Design review of the part built by this model. Coordinates are the model's own, in mm. Face numbers are marked on the shaded views. A direction names the side the tool comes from. Round coordinates to 2 decimals unless told otherwise and drop trailing zeros. Loops run counter-clockwise (first coordinate to the right, second up) from the corner with the lowest first, then second, coordinate; pieces in that order, holes last. Notation, with made-up numbers: (73, 0) - (114, 0) arc R28 cw to (114, 37) - close; hole circle Ø5 at (-12, -3.75). An arc over 180 degrees is marked (long way). Return JSON: item names as keys, results as strings. Group by question number.
from build123d import *

# Parameters (mm, degrees)
F1_DEPTH  = 20
F2_R      = 20
F3_DEPTH  = 30
F4_DEPTH  = 40
F5_W      = 33
F5_H      = 20
F6_DEPTH  = 55
F7_R      = 15
F8_DEPTH  = 20
F9_D      = 20
F11_R     = 25
F12_DEPTH = 70
F13_R     = 5


with BuildPart() as f1:
    # F0 (on Front) → F1 (new body)
    with BuildSketch(Plane.XZ):
        with BuildLine():
            ThreePointArc((-109.5042586091, -28.4546844701), (-82.4661435827, -24.3426350081), (-70, 0))
            ThreePointArc((-70, 0), (-82.4661435827, 24.3426350081), (-109.5042586091, 28.4546844701))
            ThreePointArc((-109.5042586091, 28.4546844701), (-130, 0), (-109.5042586091, -28.4546844701))
        make_face()
        with BuildLine():
            ThreePointArc((-109.5042586091, 28.4546844701), (-82.4661435827, 24.3426350081), (-70, 0))
            ThreePointArc((-70, 0), (-82.4661435827, -24.3426350081), (-109.5042586091, -28.4546844701))
            Line((-109.5042586091, -28.4546844701), (-58.6638275939, -45.4360923882))
            ThreePointArc((-58.6638275939, -45.4360923882), (-48.7715766613, -52.7166444234), (-45, -64.4058820349))
            Line((-45, -64.4058820349), (-45, -130))
            ThreePointArc((-45, -130), (-50.8578643763, -144.1421356237), (-65, -150))
            Line((-65, -150), (-80, -150))
            Line((-80, -150), (-80, -210))
            Line((-80, -210), (-60, -210))
            Line((-60, -210), (-60, -170))
            Line((-60, -170), (60, -170))
            Line((60, -170), (60, -210))
            Line((60, -210), (80, -210))
            Line((80, -210), (80, -150))
            Line((80, -150), (65, -150))
            ThreePointArc((65, -150), (50.8578643763, -144.1421356237), (45, -130))
            Line((45, -130), (45, -64.4058820349))
            ThreePointArc((45, -64.4058820349), (48.7715766613, -52.7166444234), (58.6638275939, -45.4360923882))
            Line((58.6638275939, -45.4360923882), (109.5042586091, -28.4546844701))
            ThreePointArc((109.5042586091, -28.4546844701), (70, 0), (109.5042586091, 28.4546844701))
            Line((109.5042586091, 28.4546844701), (45, 50))
            Line((45, 50), (0, 50))
            Line((0, 50), (-45, 50))
            Line((-45, 50), (-109.5042586091, 28.4546844701))
        make_face()
        with BuildLine():
            ThreePointArc((130, 0), (124.3426350081, 17.5338564173), (109.5042586091, 28.4546844701))
            ThreePointArc((109.5042586091, 28.4546844701), (70, 0), (109.5042586091, -28.4546844701))
            ThreePointArc((109.5042586091, -28.4546844701), (124.3426350081, -17.5338564173), (130, 0))
        make_face()
    extrude(amount=F1_DEPTH)

    # F2 (on face) → F3 (join)
    with BuildSketch(Plane.XZ.offset(20)):
        with Locations((100, 0)):
            Circle(F2_R)
        with Locations((-100, 0)):
            Circle(F2_R)
    extrude(amount=F3_DEPTH)

    # F2 (on face) → F4 (join)
    with BuildSketch(Plane.XZ.offset(20)):
        Polygon((-65, -150), (-80, -150), (-80, -210), (-60, -210), (-60, -170), (60, -170), (60, -210), (80, -210), (80, -150), (65, -150), align=None)
    extrude(amount=F4_DEPTH)

    # F5 (on face) → F6 (join)
    with BuildSketch(Plane.XZ.offset(60)):
        with Locations((16.5, -160)):
            Rectangle(F5_W, F5_H)
        with Locations((-16.5, -160)):
            Rectangle(F5_W, F5_H)
    extrude(amount=F6_DEPTH)

    # F7 (on face) → F8 (join)
    with BuildSketch(Plane.XZ.offset(115)):
        with BuildLine():
            ThreePointArc((-33, -227), (0, -260), (33, -227))
            ThreePointArc((33, -227), (0, -194), (-33, -227))
        make_face()
        with Locations((0, -227)):
            Circle(F7_R, mode=Mode.SUBTRACT)
        with BuildLine():
            ThreePointArc((-33, -227), (0, -194), (33, -227))
            Line((33, -227), (33, -170))
            Line((33, -170), (33, -150))
            Line((33, -150), (-33, -150))
            Line((-33, -150), (-33, -170))
            Line((-33, -170), (-33, -227))
        make_face()
    extrude(amount=F8_DEPTH)

    # F9 (through all)
    with Locations(Plane(origin=(0, 0, 0), x_dir=(1, 0, 0), z_dir=(0, 1, 0))):
        with Locations((100, 0), (-100, 0)):
            Hole(F9_D / 2)

    # F11 (on offset) → F12 (join)
    with BuildSketch(Plane.XY.offset(35)):
        with BuildLine():
            ThreePointArc((-39.9505821476, -78.0122912513), (-0.9941614801, -119.9876436284), (40, -80))
            ThreePointArc((40, -80), (39.9876436284, -79.0058385199), (39.9505821476, -78.0122912513))
            ThreePointArc((39.9505821476, -78.0122912513), (0, -40), (-39.9505821476, -78.0122912513))
        make_face()
        with Locations((0, -80)):
            Circle(F11_R, mode=Mode.SUBTRACT)
        with BuildLine():
            ThreePointArc((-39.9505821476, -78.0122912513), (0, -40), (39.9505821476, -78.0122912513))
            Line((39.9505821476, -78.0122912513), (39.9505821476, -30))
            ThreePointArc((39.9505821476, -30), (42.8795143357, -22.9289321881), (49.9505821476, -20))
            Line((49.9505821476, -20), (-49.9505821476, -20))
            ThreePointArc((-49.9505821476, -20), (-42.8795143357, -22.9289321881), (-39.9505821476, -30))
            Line((-39.9505821476, -30), (-39.9505821476, -78.0122912513))
        make_face()
    extrude(amount=-F12_DEPTH)

    # F13
    f13_edges = [f1.edges().sort_by_distance(p)[0] for p in [
        (-120, -20, 0),
        (80, -20, 0),
    ]]
    fillet(f13_edges, radius=F13_R)


solid = f1.part
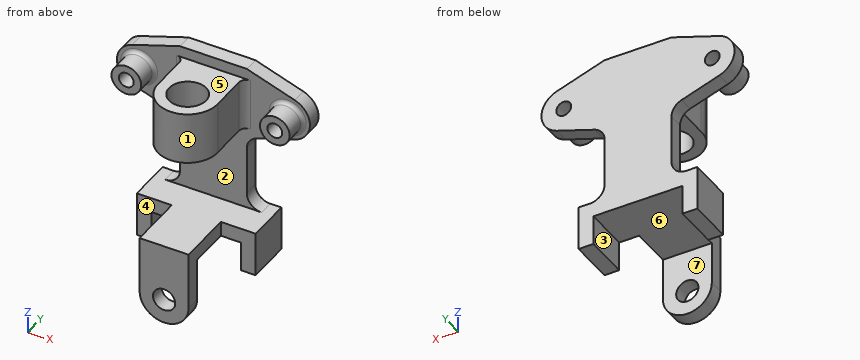
Q1. For line 1 (X direction, y = -17, z = -0.5); line 2 (Z direction, x = 39.5, y = -44.5); line 3 (Y direction, x = 0, z = 9), list the stretches that pass through material, from the lowest coordinate up.
Q2. Add section C-C, the plane x = -100. State the section outline as (y, z) points.
Q3. Add section D-D, the plane z = 4. Give the number of separate pieces and of enclosed holes in the cut face, plus the area to 3 significant figures.
Q4. Add section A-A, the plane z = -174. State the section outline as (x, y) points, plus the area to 3 significant figures.
Q5. Draft analysis for pull direction X (two halves, no side actions). For the marked faces 1, 2, 3 and 4, state which applies: pulls with the +X half, pulls with the -X half, needs draft (parallel to the pull), parting line crosses it, or undercut.
Q6. Add section B-B, the plane x = 0. State the section outline as (y, z) points.
Q7. Insertion check: pin 1 Ø14.5 at (y, z) = (-44.5, 6.5) entering from +X; pin 2 Ø6 at (x, y) = (68, -43.5) entering from -Z; pin 3 Ø3 at (x, z) = (-4.5, -103) entering from -Y. Each pin has a flat end and moves straight along its axis. Give the tip position at first contact, or say it passes through.
Q8. Tool access review of the marked faces 5, 6 and 7: name each direction out of +Z, -Z, +X, -X, +Y, -Y from which nothing blocks a thin tool from reaching the whole face with its end or side.
Evaluation:
{
 "1": {"line 1": "-130 to -109.99, -90.01 to 90.01, 109.99 to 130", "line 2": "-170 to -150, -35 to 35", "line 3": "-120 to -105, -55 to 0"},
 "2": {"outline": "(-50, -20) - (-25, -20) arc R5 cw to (-20, -25) - (-20, -31.63) - (0, -31.63) - (0, -10) - (-50, -10) - close; (-50, 10) - (0, 10) - (0, 31.63) - (-20, 31.63) - (-20, 25) arc R5 cw to (-25, 20) - (-50, 20) - close"},
 "3": {"separate pieces": "3", "enclosed holes": "1", "area": "11,100 mm²"},
 "4": {"outline": "(-80, -60) - (-60, -60) - (-60, 0) - (-80, 0) - close; (-33, -135) - (33, -135) - (33, -115) - (-33, -115) - close; (60, -60) - (80, -60) - (80, 0) - (60, 0) - close", "area": "3,720 mm²"},
 "5": {"face 1": "parting line crosses it", "face 2": "undercut", "face 3": "undercut", "face 4": "needs draft"},
 "6": {"outline": "(-135, -260) - (-115, -260) - (-115, -242) - (-135, -242) - close; (-135, -212) - (-115, -212) - (-115, -170) - (0, -170) - (0, 50) - (-20, 50) - (-20, 35) - (-55, 35) - (-55, -35) - (-20, -35) - (-20, -150) - (-135, -150) - close; (-120, -35) - (-105, -35) - (-105, 35) - (-120, 35) - close"},
 "7": {"pin 1": "x = 120", "pin 2": "z = -210", "pin 3": "y = -20"},
 "8": {"face 5": "+Z, +X, -X, -Y", "face 6": "-Z, +Y", "face 7": "-Z, +X, -X, +Y"}
}
